Part model, mm, in its own coordinate system. Round coordinates to 2 decimals unless told otherwise and drop trailing zeros. Write each loop counter-clockwise with the first axis right and the second up, starting at its lowest first coordinate (ties: lowest second). Pieces come first, ordered by that corner, then holes. Notation, with made-up numbers: (63, -33) -> (67, -33) arc R23 ccw to (67, -2) -> close; hole circle Ø10 at (47.25, 55). An arc over 180 degrees is marked (long way). Use CSV: the item, a comma, the result in double quotes. Start each with the question number.
(1) Saw through at D-D (z = -15). Give the cut face in (x, y) (3 decimals), plus the area to 3 significant figures.
(2) Drop flat-ended pins along their axis: pin 1 (1.9 mm diameter, centred on x = -25, z = -7.5, fed in from +Y); pin 2 (4 mm diameter, centred on x = 25, z = 7.5, fed in from +Y) (3 decimals). Give the stop position or say it passes through.
(3) Saw through at A-A (y = 0.55). Give the cut face in (x, z).
(4) Saw through at C-C (x = 25). Give the cut face in (y, z) (3 decimals).
(5) Probe line 1 (X direction, y = 0.7, z = 7.5); line 2 (Z direction, x = -24.5, y = 0.65); line 3 (X direction, y = 2.5, z = 14). List the from-to ranges inside material, lowest first. Write a range as [from, to].
(6) Saw through at B-B (z = -7.5). Give the cut face in (x, y) (3 decimals), plus the area to 3 significant figures.
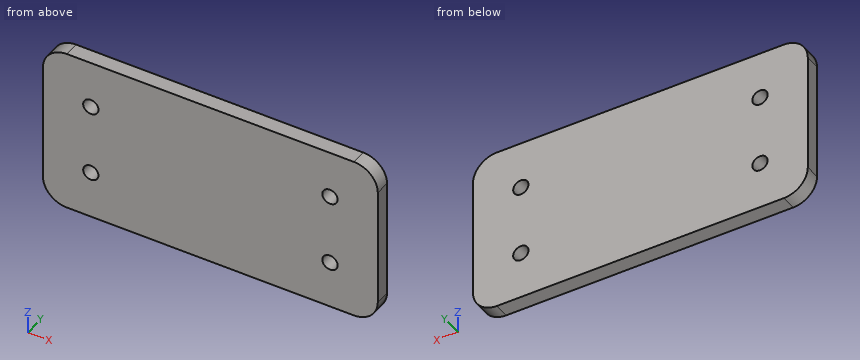
```python
from build123d import *

# Parameters (mm, degrees)
SKETCH1_W           = 70
SKETCH1_H           = 35
BOSS_EXTRUDE1_DEPTH = 3.175
SKETCH2_R           = 1.6
CUT_EXTRUDE1_DEPTH  = 3.175
FILLET1_R           = 5


with BuildPart() as part:
    # Sketch1 → Boss-Extrude1 (new body)
    with BuildSketch(Plane(origin=(0, 0, 0), x_dir=(1, 0, 0), z_dir=(0, 1, 0))):
        Rectangle(SKETCH1_W, SKETCH1_H)
    extrude(amount=BOSS_EXTRUDE1_DEPTH)

    # Sketch2 → Cut-Extrude1 (cut)
    with BuildSketch(Plane(origin=(0, 3.175, 0), x_dir=(1, 0, 0), z_dir=(0, 1, 0))):
        with Locations(Location((-25, 7.5, 0), (0, 0, 270))):
            Circle(SKETCH2_R)
        with Locations(Location((-25, -7.5, 0), (0, 0, 270))):
            Circle(SKETCH2_R)
        with Locations(Location((25, -7.5, 0), (0, 0, 270))):
            Circle(SKETCH2_R)
        with Locations(Location((25, 7.5, 0), (0, 0, 270))):
            Circle(SKETCH2_R)
    extrude(amount=-CUT_EXTRUDE1_DEPTH, mode=Mode.SUBTRACT)

    # Fillet1
    fillet1_edges = [part.edges().sort_by_distance(p)[0] for p in [
        (35, 1.5875, 17.5),
        (-35, 1.5875, 17.5),
        (-35, 1.5875, -17.5),
        (35, 1.5875, -17.5),
    ]]
    fillet(fillet1_edges, radius=FILLET1_R)


solid = part.part
```
Answers:
1,outline,"(-34.33, 0) -> (34.33, 0) -> (34.33, 3.175) -> (-34.33, 3.175) -> close"
1,area,"218 mm²"
2,pin 1,"passes through"
2,pin 2,"stops at y = 3.175"
3,outline,"(-35, -12.5) arc R5 ccw to (-30, -17.5) -> (30, -17.5) arc R5 ccw to (35, -12.5) -> (35, 12.5) arc R5 ccw to (30, 17.5) -> (-30, 17.5) arc R5 ccw to (-35, 12.5) -> close; hole circle Ø3.2 at (-25, -7.5); hole circle Ø3.2 at (-25, 7.5); hole circle Ø3.2 at (25, -7.5); hole circle Ø3.2 at (25, 7.5)"
4,outline,"(0, -17.5) -> (3.175, -17.5) -> (3.175, -9.1) -> (0, -9.1) -> close; (0, -5.9) -> (3.175, -5.9) -> (3.175, 5.9) -> (0, 5.9) -> close; (0, 9.1) -> (3.175, 9.1) -> (3.175, 17.5) -> (0, 17.5) -> close"
5,line 1,"x = [-35, -26.6], [-23.4, 23.4], [26.6, 35]"
5,line 2,"z = [-17.5, -9.02], [-5.98, 5.98], [9.02, 17.5]"
5,line 3,"x = [-34.77, 34.77]"
6,outline,"(-35, 0) -> (-26.6, 0) -> (-26.6, 3.175) -> (-35, 3.175) -> close; (-23.4, 0) -> (23.4, 0) -> (23.4, 3.175) -> (-23.4, 3.175) -> close; (26.6, 0) -> (35, 0) -> (35, 3.175) -> (26.6, 3.175) -> close"
6,area,"202 mm²"
